Can you work these out from the model? Positions are in its coordinate system, mm. A direction names the side the tool comes from. Coordinates: 2 decimals unless noted, no trailing zeros. Write each loop counter-clockwise with the first axis right and the second up, starting at its lowest first coordinate (ties: lowest second). Pieces come first, ordered by that corner, then holes. Notation, with made-up numbers: (-6.75, -12) - (14.25, -12) arc R11 cw to (14.25, 8) - close; hole circle Ø7 at (44, -39). An arc over 180 degrees is marked (long way). Use one line per item in the form item = value. Start each with the question number.
(1) For pin 1 Ø16 at (x, z) = (79, -50.5) entering from +Y; pin 2 Ø12 at (y, z) = (22, -79) entering from -X, each with a flat end and sliding along its axis, tell me the tip position at first contact or that it passes through.
(2) Thinking about a two-plate mould opening in Z: for faces 1 (the face through (50, 50, -101.6)), 2 (the face through (29, 98.1, -21)), 3 (the face through (98.1, 21, -29)), 4 (the face through (84.37, 91.41, -99.87)), which applies, pulls with the +Z half, pulls with the -Z half, needs draft (parallel to the pull), parting line crosses it, or undercut?
(3) If we section it at B-B on z = -90: Please give me the cut outline in (x, y), then the cut area to 3 significant figures.
(4) If we section it at D-D on z = -26: Please give me the cut outline in (x, y).
(5) On a 3-axis mill with a long thin cutter (end or side, diameter ignored), from which of +Z, -Z, +X, -X, +Y, -Y can I reach the whole of each face in a straight line? I mean faces 5 (the face through (26.861, 96.418, -1.726)), 6 (the face through (98.1, 51, -80)), 7 (the face through (29, 98.1, -81)), 8 (the face through (11.262, 1.726, -38.202)). Say none if no direction works.
(6) If we section it at A-A on y = 50.8: Please give me the cut outline in (x, z), then the cut area to 3 significant figures.
(7) If we section it at C-C on x = 61: Please give me the cut outline in (y, z).
(8) If I drill on probe 1 along Z at (x, y) = (99, 50); probe 2 along X at (y, z) = (2, -50); probe 3 along X at (y, z) = (60, -13), over which ranges is the centre line in solid material (lowest first)? Write a range as from..to.
```python
from build123d import *

# Parameters (mm, degrees)
SKETCH1_W           = 101.6
SKETCH1_H           = 101.6
BOSS_EXTRUDE2_DEPTH = 101.6
SKETCH3_R           = 15.875
CUT_EXTRUDE1_DEPTH  = 3.500000112
SKETCH4_R           = 15.875
CUT_EXTRUDE2_DEPTH  = 3.500000112
SKETCH5_R           = 15.875
CUT_EXTRUDE3_DEPTH  = 3.500000112
SKETCH6_R           = 15.875
CUT_EXTRUDE4_DEPTH  = 3.500000112
SKETCH7_R           = 15.875
CUT_EXTRUDE5_DEPTH  = 3.500000112
SKETCH8_R           = 15.875
CUT_EXTRUDE6_DEPTH  = 3.500000112


with BuildPart() as part:
    # Sketch1 → Boss-Extrude2 (new body)
    with BuildSketch(Plane(origin=(0, 0, 0), x_dir=(1, 0, 0), z_dir=(0, 1, 0))):
        with Locations((50.8, 50.8)):
            Rectangle(SKETCH1_W, SKETCH1_H)
    extrude(amount=BOSS_EXTRUDE2_DEPTH)

    # Sketch3 → Cut-Extrude1 (cut)
    with BuildSketch(Plane(origin=(0, 101.6, 0), x_dir=(1, 0, 0), z_dir=(0, 1, 0))):
        with Locations(Location((28.927876431, 20.922123569, 0), (0, 0, 270))):
            Circle(SKETCH3_R)
        with Locations(Location((28.927876431, 80.677876431, 0), (0, 0, 270))):
            Circle(SKETCH3_R)
        with Locations(Location((80.677876431, 50.8, 0), (0, 0, 270))):
            Circle(SKETCH3_R)
    extrude(amount=-CUT_EXTRUDE1_DEPTH, mode=Mode.SUBTRACT)

    # Sketch4 → Cut-Extrude2 (cut)
    with BuildSketch(Plane.ZY):
        with Locations((-72.672123569, 20.922123569)):
            Circle(SKETCH4_R)
        with Locations((-72.672123569, 80.677876431)):
            Circle(SKETCH4_R)
        with Locations((-20.922123569, 50.8)):
            Circle(SKETCH4_R)
    extrude(amount=-CUT_EXTRUDE2_DEPTH, mode=Mode.SUBTRACT)

    # Sketch5 → Cut-Extrude3 (cut)
    with BuildSketch(Plane(origin=(0, 0, -101.6), x_dir=(-1, 0, 0), z_dir=(0, 0, -1))):
        with Locations((-72.672123569, 20.922123569)):
            Circle(SKETCH5_R)
        with Locations((-72.672123569, 80.677876431)):
            Circle(SKETCH5_R)
        with Locations((-20.922123569, 50.8)):
            Circle(SKETCH5_R)
    extrude(amount=-CUT_EXTRUDE3_DEPTH, mode=Mode.SUBTRACT)

    # Sketch6 → Cut-Extrude4 (cut)
    with BuildSketch(Plane(origin=(101.6, 0, 0), x_dir=(0, 0, -1), z_dir=(1, 0, 0))):
        with Locations((28.927876431, 20.922123569)):
            Circle(SKETCH6_R)
        with Locations((28.927876431, 80.677876431)):
            Circle(SKETCH6_R)
        with Locations((80.677876431, 50.8)):
            Circle(SKETCH6_R)
    extrude(amount=-CUT_EXTRUDE4_DEPTH, mode=Mode.SUBTRACT)

    # Sketch7 → Cut-Extrude5 (cut)
    with BuildSketch(Plane.XY):
        with Locations((28.927876431, 20.922123569)):
            Circle(SKETCH7_R)
        with Locations((28.927876431, 80.677876431)):
            Circle(SKETCH7_R)
        with Locations((80.677876431, 50.8)):
            Circle(SKETCH7_R)
    extrude(amount=-CUT_EXTRUDE5_DEPTH, mode=Mode.SUBTRACT)

    # Sketch8 → Cut-Extrude6 (cut)
    with BuildSketch(Plane(origin=(0, 0, 0), x_dir=(-1, 0, 0), z_dir=(0, -1, 0))):
        with Locations(Location((-72.672123569, 20.922123569, 0), (0, 0, 90))):
            Circle(SKETCH8_R)
        with Locations(Location((-72.672123569, 80.677876431, 0), (0, 0, 90))):
            Circle(SKETCH8_R)
        with Locations(Location((-20.922123569, 50.8, 0), (0, 0, 90))):
            Circle(SKETCH8_R)
    extrude(amount=-CUT_EXTRUDE6_DEPTH, mode=Mode.SUBTRACT)


solid = part.part
```
Reported:
q1.pin_1 = 98.1
q1.pin_2 = 3.5
q2.face_1 = pulls with the -Z half
q2.face_2 = undercut
q2.face_3 = undercut
q2.face_4 = needs draft
q3.outline = (0, 0) - (59.82, 0) - (59.82, 3.5) - (85.52, 3.5) - (85.52, 0) - (101.6, 0) - (101.6, 37.95) - (98.1, 37.95) - (98.1, 63.65) - (101.6, 63.65) - (101.6, 101.6) - (41.78, 101.6) - (41.78, 98.1) - (16.08, 98.1) - (16.08, 101.6) - (0, 101.6) - close
q3.area = 10,100 mm2
q4.outline = (0, 0) - (57.63, 0) - (57.63, 3.5) - (87.71, 3.5) - (87.71, 0) - (101.6, 0) - (101.6, 5.32) - (98.1, 5.32) - (98.1, 36.52) - (101.6, 36.52) - (101.6, 65.08) - (98.1, 65.08) - (98.1, 96.28) - (101.6, 96.28) - (101.6, 101.6) - (43.97, 101.6) - (43.97, 98.1) - (13.89, 98.1) - (13.89, 101.6) - (0, 101.6) - (0, 65.84) - (3.5, 65.84) - (3.5, 35.76) - (0, 35.76) - close
q5.face_5 = +Z
q5.face_6 = +X
q5.face_7 = +Y
q5.face_8 = -Y
q6.outline = (0, -101.6) - (5.05, -101.6) - (5.05, -98.1) - (36.8, -98.1) - (36.8, -101.6) - (101.6, -101.6) - (101.6, -96.55) - (98.1, -96.55) - (98.1, -64.8) - (101.6, -64.8) - (101.6, 0) - (96.55, 0) - (96.55, -3.5) - (64.8, -3.5) - (64.8, 0) - (0, 0) - (0, -5.05) - (3.5, -5.05) - (3.5, -36.8) - (0, -36.8) - close
q6.area = 9,880 mm2
q7.outline = (0, -101.6) - (10.16, -101.6) - (10.16, -98.1) - (31.68, -98.1) - (31.68, -101.6) - (69.92, -101.6) - (69.92, -98.1) - (91.44, -98.1) - (91.44, -101.6) - (101.6, -101.6) - (101.6, 0) - (0, 0) - (0, -10.16) - (3.5, -10.16) - (3.5, -31.68) - (0, -31.68) - (0, -69.92) - (3.5, -69.92) - (3.5, -91.44) - (0, -91.44) - close
q8.probe_1 = -101.6..-96.53, -64.82..0
q8.probe_2 = 0..5.07, 36.78..101.6
q8.probe_3 = 3.5..101.6
